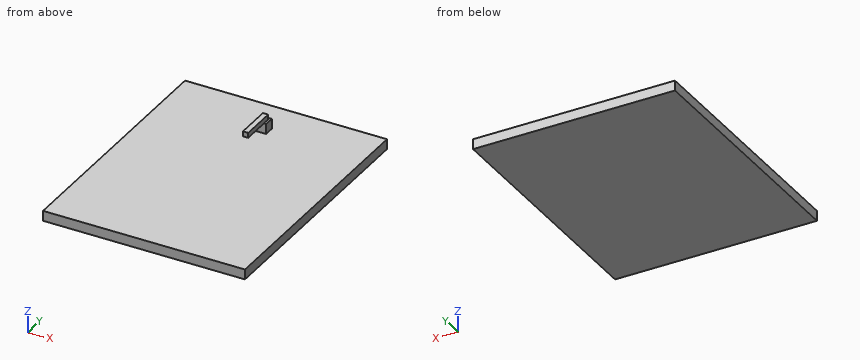
```python
from build123d import *

# Parameters (mm, degrees)
F0_W     = 200
F0_H     = 250
F1_DEPTH = 10
F2_W     = 5.21805
F2_H     = 10
F2_W_2   = 4.78195
F3_DEPTH = 10
F5_W     = 5.184704
F5_H     = 5.141512
F6_DEPTH = 5
F7_W     = 5.184704
F7_H     = 5
F8_DEPTH = 30


with BuildPart() as f1:
    # F0 (on Top) → F1 (new body)
    with BuildSketch(Plane.XY):
        Rectangle(F0_W, F0_H)
    extrude(amount=F1_DEPTH)

    # F2 (on face) → F3 (join)
    with BuildSketch(Plane.XY.offset(10)):
        with Locations((-2.609025, 86.457404)):
            Rectangle(F2_W, F2_H)
        with Locations((2.390975, 86.457404)):
            Rectangle(F2_W_2, F2_H)
    extrude(amount=F3_DEPTH)

    # F5 (on face) → F6 (join)
    with BuildSketch(Plane.XY.offset(20)):
        with Locations((0, 86.392045)):
            Rectangle(F5_W, F5_H)
    extrude(amount=F6_DEPTH)

    # F7 (on face) → F8 (join)
    with BuildSketch(Plane.XZ.offset(-83.821289)):
        with Locations((0, 22.5)):
            Rectangle(F7_W, F7_H)
    extrude(amount=F8_DEPTH)


solid = f1.part
```
Geometry check sheet. Reference: the model listing, model coordinates, mm. Coordinates: 2 decimals unless noted, no trailing zeros. Loops run counter-clockwise (first coordinate to the right, second up) from the corner with the lowest first, then second, coordinate; pieces in that order, holes last.
Item 1: Sectioned sample at B-B, the plane x = -63. Record the boundary of the cut face in (y, z), then the cut area to 3 significant figures.
Item 2: Thickness scan on line 1 (Z direction, x = -72.5, y = 94.5); line 2 (Y direction, x = -3.5, z = 14). Record the ranges inside material, lowest first.
Item 3: Sectioned sample at A-A, the plane y = 68. Record the boundary of the cut face in (x, z).
Item 4: Go/stop test with flat-tipped pins: pin 1 Ø5.5 at (y, z) = (64.5, 22) entering from +X; pin 2 Ø2 at (x, y) = (52, -3) entering from +Z; pin 3 Ø11 at (y, z) = (87.5, 17.5) entering from +X. Record where each tip stops, or that it passes through.
Item 5: Sectioned sample at C-C, the plane y = -48.5. Record the boundary of the cut face in (x, z), then the cut area to 3 significant figures.
Check result:
1. outline: (-125, 0) - (125, 0) - (125, 10) - (-125, 10) - close
1. area: 2,500 mm2
2. line 1: z = 0 to 10
2. line 2: y = 81.46 to 91.46
3. outline: (-100, 0) - (100, 0) - (100, 10) - (-100, 10) - close; (-2.59, 20) - (2.59, 20) - (2.59, 25) - (-2.59, 25) - close
4. pin 1: stops at x = 2.59
4. pin 2: stops at z = 10
4. pin 3: stops at x = 4.78
5. outline: (-100, 0) - (100, 0) - (100, 10) - (-100, 10) - close
5. area: 2,000 mm2
